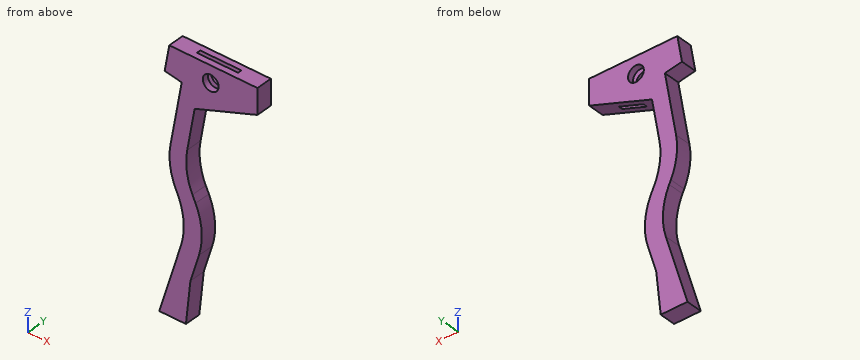
```python
from build123d import *

# Parameters (mm, degrees)
F1_DEPTH = 30
F2_R     = 250
F3_R     = 29.586719
F4_DEPTH = 60.001
F5_R     = 100
F6_DEPTH = 7.5


with BuildPart() as f1:
    # F0 (on Front) → F1 (new body, symmetric)
    with BuildSketch(Plane.XZ):
        Polygon((-79.632452, 408.511814), (-15.619948, 397.224683), (-71.23988, 81.788369), (8.866352, -90), (-100, -448.849714), (0, -448.849714), (16.78813, -289.121331), (76.358088, -92.764401), (0, 70.986047), (-8.866352, 90), (0, 140.283579), (32.809211, 326.353861), (267.732366, 411.858897), (267.732366, 506.99259), (-62.267634, 506.99259), align=None)
    extrude(amount=F1_DEPTH, both=True)

    # F2
    f2_edges = [f1.edges().sort_by_distance(p)[0] for p in [
        (-8.866352, 0, 90),
        (76.358088, 0, -92.764401),
        (-71.23988, 0, 81.788369),
        (8.866352, 0, -90),
    ]]
    fillet(f2_edges, radius=F2_R)

    # F3 (on face) → F4 (cut, through all)
    with BuildSketch(Plane.XZ.offset(30)):
        with Locations((92.837751, 444.634497)):
            Circle(F3_R)
    extrude(amount=-F4_DEPTH, mode=Mode.SUBTRACT)

    # F5 (on Front) → F6 (cut, symmetric)
    with BuildSketch(Plane.XZ):
        with Locations((99.455066, 443.239033)):
            Circle(F5_R)
    extrude(amount=F6_DEPTH, both=True, mode=Mode.SUBTRACT)


solid = f1.part
```
Input: part model. Units: mm. Frame: model coordinates. Give positions to 0.01 mm unless a question says otherwise; leave off trailing zeros. Order: outer loops, then holes, each group sorted by start corner. A loop starts at its lowest first (then second) coordinate and runs counter-clockwise, first axis right, second up. Notation, with made-up numbers: M 38.5,-20.5 L 65.5,-20.5 A17 ccw 65.5,-10.5 Z; hole C 57,1 d10. An arc over 180 degrees is marked long. One line per question, with ' | ' between items.
1) Ray query, L1, parallel to Y at x = 69, z = 385; L2, parallel to X at y = 19, z = -111.5; L3, parallel to X at y = -27, z = 464. Return the intervals inside material, ascending.
Filled in:
L1: y = -30 to -7.5, 7.5 to 30 | L2: x = -8.15 to 59.35 | L3: x = -69.85 to 70.47, 115.21 to 267.73
2) Section C-C on x = 242. Output: boundary loops of the cut face in (y, z), and give its area (3 significant figures).
Filled in:
outline: M -30,402.49 L 30,402.49 L 30,506.99 L -30,506.99 Z | area: 6,270 mm2
3) Section A-A on x = 93. Output: boundary loops of the cut face in (y, z).
Filled in:
outline: M -30,348.26 L -7.5,348.26 L -7.5,415.05 L -30,415.05 Z; M -30,474.22 L -7.5,474.22 L -7.5,506.99 L -30,506.99 Z; M 7.5,348.26 L 30,348.26 L 30,415.05 L 7.5,415.05 Z; M 7.5,474.22 L 30,474.22 L 30,506.99 L 7.5,506.99 Z
4) Section B-B on z = 234.5. Output: boundary loops of the cut face in (x, y).
Filled in:
outline: M -44.31,-30 L 16.61,-30 L 16.61,30 L -44.31,30 Z
5) Contact query for flat-ended pins moving along their axis: P1, Ø2, axis at y = -10, z = -70.5, coming from the -X side; P2, Ø3, axis at x = 78, y = -7.5, coming from the -Z side; P3, Ø5, axis at y = -7.5, z = 99.5, coming from the -X side. Output: stop coordinate, or through.
Filled in:
P1: stops at x = -11.27 | P2: stops at z = 342.26 | P3: stops at x = -60.96
